Source: CAD feature listing. Evaluate the final solid. Frame: model axes, mm. Face numbers are marked on the shaded views. A direction names the side the tool comes from. Round coordinates to 2 decimals unless told otherwise and drop trailing zeros. Write each loop counter-clockwise with the first axis right and the second up, starting at its lowest first coordinate (ties: lowest second). Pieces come first, ordered by that corner, then holes. Notation, with made-up numbers: M 53.5,-12.75 L 57.5,-12.75 A5 cw 57.5,-6.75 Z; hole C 18.5,44.5 d1. An arc over 180 degrees is marked long. Answer in a Markdown table with one row per item.
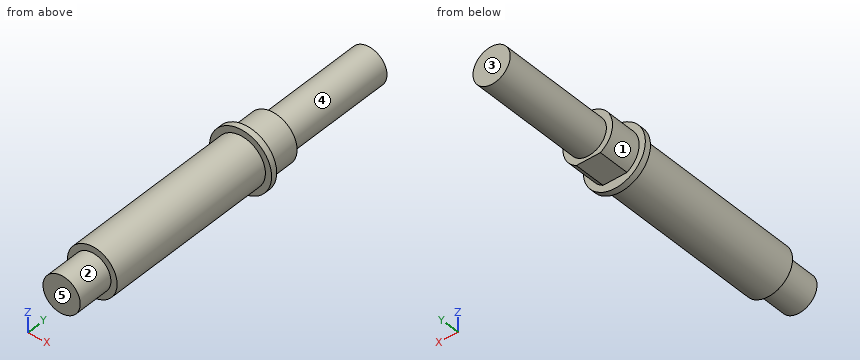
from build123d import *

# Parameters (mm, degrees)
SKETCH_1_R      = 1.5
EXTRUDE_1_DEPTH = 30
EXTRUDE_START   = 15
SKETCH_2_R      = 2
SKETCH_2_R_2    = 1.5
EXTRUDE_2_DEPTH = 15
SKETCH_3_R      = 1.5
EXTRUDE_3_DEPTH = 2.6
EXTRUDE_START_2 = -0.5
SKETCH_4_R      = 2.5
SKETCH_4_R_2    = 2
EXTRUDE_4_DEPTH = 0.5


with BuildPart() as part:
    # 草图1 → 凸台-拉伸1 (new body)
    with BuildSketch(Plane(origin=(0, 0, 0), x_dir=(1, 0, 0), z_dir=(0, 1, 0))):
        with Locations(Location((0, 0, 0), (0, 0, 270))):
            Circle(SKETCH_1_R)
    extrude(amount=EXTRUDE_1_DEPTH)

    # 草图2 → 凸台-拉伸2 (add)
    with BuildSketch(Plane(origin=(0, 18, 0), x_dir=(-1, 0, 0), z_dir=(0, -1, 0)).offset(EXTRUDE_START)):
        with Locations(Location((0, 0, 0), (0, 0, 90))):
            Circle(SKETCH_2_R)
        with Locations(Location((0, 0, 0), (0, 0, 90))):
            Circle(SKETCH_2_R_2, mode=Mode.SUBTRACT)
    extrude(amount=-EXTRUDE_2_DEPTH)

    # 草图3 → 凸台-拉伸3 (add)
    with BuildSketch(Plane(origin=(0, 18, 0), x_dir=(1, 0, 0), z_dir=(0, 1, 0))):
        with BuildLine():
            Line((0.91625301, 1.777774007), (-1.022249701, 1.719012958))
            ThreePointArc((-1.022249701, 1.719012958), (0.060597358, -1.999081779), (0.91625301, 1.777774007))
        make_face()
        with Locations(Location((0, 0, 0), (0, 0, 90))):
            Circle(SKETCH_3_R, mode=Mode.SUBTRACT)
    extrude(amount=EXTRUDE_3_DEPTH)

    # 草图4 → 凸台-拉伸4 (add)
    with BuildSketch(Plane(origin=(0, 18, 0), x_dir=(1, 0, 0), z_dir=(0, 1, 0)).offset(EXTRUDE_START_2)):
        with Locations(Location((0, 0, 0), (0, 0, 270))):
            Circle(SKETCH_4_R)
        with Locations(Location((0, 0, 0), (0, 0, 270))):
            Circle(SKETCH_4_R_2, mode=Mode.SUBTRACT)
    extrude(amount=EXTRUDE_4_DEPTH)


solid = part.part
Q1. Access query for the marked faces 1, 2 and 3. Directions: +Z, -Z, +X, -X, +Y, -Y. A direction counts if a zero-diameter tool reaches every point of the face in a straight line with its end or side. Return the directions, or none.
Solutions:
| item | result |
|---|---|
| face 1 | +Y |
| face 2 | -Y |
| face 3 | +Z, -Z, +X, -X, +Y |
Q2. Section C-C (y = 4). Return loops of the section in (x, z), and give its area (3 significant figures).
Solutions:
| item | result |
|---|---|
| outline | C 0,0 d4 |
| area | 12.6 mm2 |
Q3. Contact query for a flat-ended pin moving along its axis: pin 1 Ø1.5 at (y, z) = (20.5, 0) entering from -X. Output: stop coordinate, or through.
Solutions:
| item | result |
|---|---|
| pin 1 | stops at x = -2 |
Q4. Section A-A (x = 0). Return loops of the section in (y, z).
Solutions:
| item | result |
|---|---|
| outline | M 0,-1.5 L 3,-1.5 L 3,-2 L 17.5,-2 L 17.5,-2.5 L 18,-2.5 L 18,-1.75 L 20.6,-1.75 L 20.6,-1.5 L 30,-1.5 L 30,1.5 L 20.6,1.5 L 20.6,2 L 18,2 L 18,2.5 L 17.5,2.5 L 17.5,2 L 3,2 L 3,1.5 L 0,1.5 Z |
Q5. Material intervals for probe 1 along Y at (x, z) = (1.7, -1.35); probe 2 along Y at (x, z) = (-0.4, 1.9); probe 3 along Z at (x, y) = (0.1, 17.75), sorted ascending.
Solutions:
| item | result |
|---|---|
| probe 1 | y = 17.5 to 18 |
| probe 2 | y = 3 to 20.6 |
| probe 3 | z = -2.5 to 2.5 |
Q6. Section D-D (y = 25). Return loops of the section in (x, z).
Solutions:
| item | result |
|---|---|
| outline | C 0,0 d3 |
Q7. Section B-B (z = 0). Return loops of the section in (x, y).
Solutions:
| item | result |
|---|---|
| outline | M -2.5,17.5 L -2,17.5 L -2,3 L -1.5,3 L -1.5,0 L 1.5,0 L 1.5,3 L 2,3 L 2,17.5 L 2.5,17.5 L 2.5,18 L 2,18 L 2,20.6 L 1.5,20.6 L 1.5,30 L -1.5,30 L -1.5,20.6 L -2,20.6 L -2,18 L -2.5,18 Z |
Q8. Pull-direction query (X, two-part tool) for the marked faces 4 and 5; classes: pulls with the +X half, pulls with the -X half, needs draft (parallel to the pull), parting line crosses it, or undercut.
Solutions:
| item | result |
|---|---|
| face 4 | parting line crosses it |
| face 5 | needs draft |
